The drawing under review shows one solid part. Ordinate dimensions are in mm from its lowest x, y, z. Give positions to 0.01 mm unless a question says otherwise; leave off trailing zeros. Write each loop counter-clockwise with the first axis right and the second up, starting at its lowest first coordinate (ties: lowest second). Pieces come first, ordered by that corner, then holes. Notation, with made-up numbers: (15, 15) -> (47, 15) arc R26 cw to (47, 44) -> close; hole circle Ø10 at (-2, 36.25). An arc over 180 degrees is marked (long way). Write item = value, one per line.
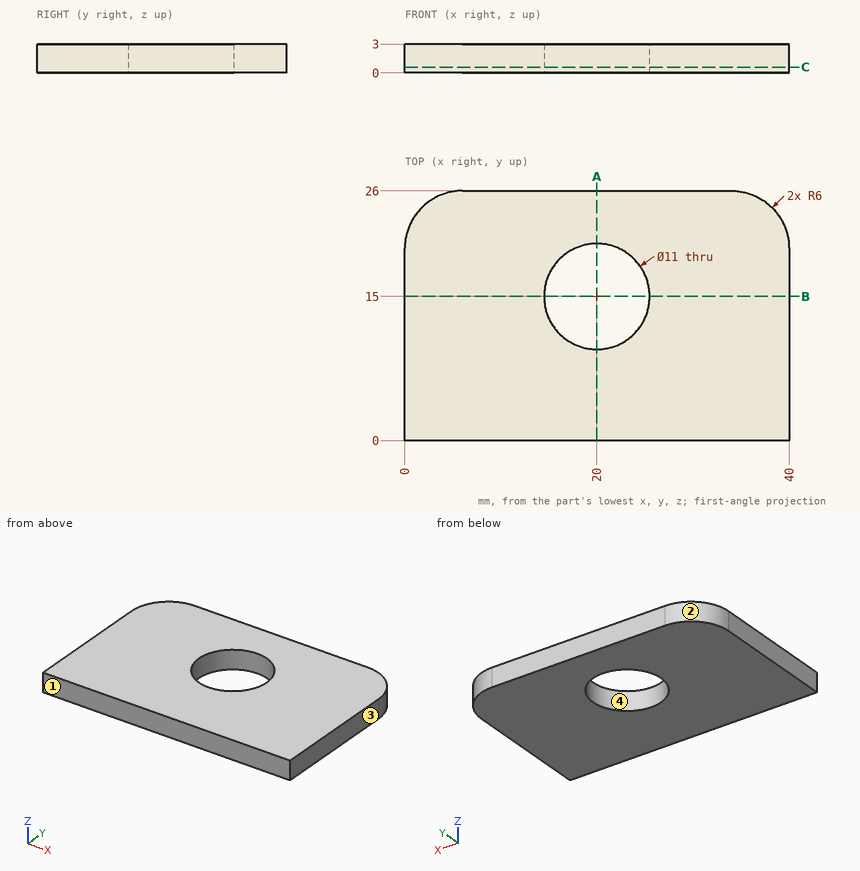
(1) Take a section at A-A (x = 20). Write out the cut boundary in (y, z), plus the area to 3 significant figures.
Answers below:
outline = (0, 0) -> (9.5, 0) -> (9.5, 3) -> (0, 3) -> close; (20.5, 0) -> (26, 0) -> (26, 3) -> (20.5, 3) -> close
area = 45.0 mm^2
(2) Take a section at B-B (y = 15). Write out the cut boundary in (x, z), plus the area to 3 significant figures.
Answers below:
outline = (0, 0) -> (14.5, 0) -> (14.5, 3) -> (0, 3) -> close; (25.5, 0) -> (40, 0) -> (40, 3) -> (25.5, 3) -> close
area = 87.0 mm^2
(3) The part is to be moulded in two halves that separate along Y. For the marked faces 1, 2, 3 and 4, say which applies: released by +Y, released by -Y, zero draft, split by the parting line, or undercut.
Answers below:
face_1 = released by -Y
face_2 = released by +Y
face_3 = zero draft
face_4 = undercut
(4) Take a section at C-C (z = 0.6). Write out the cut boundary in (x, y).
Answers below:
outline = (0, 0) -> (40, 0) -> (40, 20) arc R6 ccw to (34, 26) -> (6, 26) arc R6 ccw to (0, 20) -> close; hole circle Ø11 at (20, 15)
(5) To check wall thickness, follow probe 1 along Y at (x, z) = (20, 1.7); probe 2 along X at (y, z) = (16.75, 0.75); probe 3 along X at (y, z) = (14.5, 0.5). State the ranges of each line that lie inside material, in increasing order.
Answers below:
probe_1 = 0 to 9.5, 20.5 to 26
probe_2 = 0 to 14.79, 25.21 to 40
probe_3 = 0 to 14.52, 25.48 to 40
